from build123d import *

# Parameters (mm, degrees)
SKETCH_1_W          = 29.00004826
SKETCH_1_H          = 8.2
EXTRUDE_1_DEPTH     = 1
SKETCH_3_W          = 24.987345695
SKETCH_3_H          = 8.2
EXTRUDE_2_DEPTH     = 1
SKETCH_4_W          = 27.987350775
SKETCH_4_H          = 8.2
EXTRUDE_3_DEPTH     = 1
SKETCH_6_W          = 23.983586282
SKETCH_6_H          = 8.2
EXTRUDE_4_DEPTH     = 1
SKETCH_9_W          = 12.5
SKETCH_9_H          = 4.4
CUT_EXTRUDE_1_DEPTH = 1
SKETCH_10_W         = 29.00004826
SKETCH_10_H         = 25.974648209
EXTRUDE_5_DEPTH     = 1
SKETCH_11_W         = 13.604013208
SKETCH_11_H         = 7
CUT_EXTRUDE_3_DEPTH = 1
FILLET_1_R          = 1
FILLET_2_R          = 1
CUT_EXTRUDE_START   = -8.200051
SKETCH_12_W         = 27.27465329
SKETCH_12_H         = 24.274648209
SKETCH_12_W_2       = 26.97465329
SKETCH_12_H_2       = 23.974648209
CUT_EXTRUDE_4_DEPTH = 8.200051
EXTRUDE_START       = -5.1e-05
SKETCH_14_W         = 0.8
SKETCH_14_H         = 0.8
EXTRUDE_6_DEPTH     = 2
FILLET_3_R          = 0.8


# Some blends are built 0.0001 mm under size
with BuildPart() as part:
    # 草图1 → 凸台-拉伸1 (new body)
    with BuildSketch(Plane.XY):
        with Locations((-13.373026416, 0.4999492)):
            Rectangle(SKETCH_1_W, SKETCH_1_H)
    extrude(amount=EXTRUDE_1_DEPTH)

    # 草图3 → 凸台-拉伸2 (add)
    with BuildSketch(Plane.ZY.offset(26.860353061)):
        with Locations((-12.493672848, 0.4999492)):
            Rectangle(SKETCH_3_W, SKETCH_3_H)
    extrude(amount=EXTRUDE_2_DEPTH)

    # 草图4 → 凸台-拉伸3 (add)
    with BuildSketch(Plane(origin=(0, 0, -23.974648209), x_dir=(-1, 0, 0), z_dir=(0, 0, -1))):
        with Locations((12.866677673, 0.4999492)):
            Rectangle(SKETCH_4_W, SKETCH_4_H)
    extrude(amount=EXTRUDE_3_DEPTH)

    # 草图6 → 凸台-拉伸4 (add)
    with BuildSketch(Plane(origin=(0.114300229, 0, 0), x_dir=(0, 0, -1), z_dir=(1, 0, 0))):
        with Locations((11.991793141, 0.5)):
            Rectangle(SKETCH_6_W, SKETCH_6_H)
    extrude(amount=EXTRUDE_4_DEPTH)

    # 草图9 → 切除-拉伸1 (cut)
    with BuildSketch(Plane(origin=(1.114300229, 0, 0), x_dir=(0, 0, -1), z_dir=(1, 0, 0))):
        with Locations((11.541221742, 2.4)):
            Rectangle(SKETCH_9_W, SKETCH_9_H)
    extrude(amount=-CUT_EXTRUDE_1_DEPTH, mode=Mode.SUBTRACT)

    # 草图10 → 凸台-拉伸5 (add)
    with BuildSketch(Plane.XZ.offset(3.6)):
        with Locations((-13.373026416, -11.987324105)):
            Rectangle(SKETCH_10_W, SKETCH_10_H)
    extrude(amount=EXTRUDE_5_DEPTH)

    # 草图11 → 切除-拉伸3 (cut)
    with BuildSketch(Plane.XZ.offset(4.6)):
        with Locations((-15.621031242, -16.494333249)):
            Rectangle(SKETCH_11_W, SKETCH_11_H)
    extrude(amount=-CUT_EXTRUDE_3_DEPTH, mode=Mode.SUBTRACT)

    # 圆角1
    fillet_1_edges = [part.edges().sort_by_distance(p)[0] for p in [
        (1.126997714, -2.54e-05, -24.974648209),
        (1.126997714, -2.54e-05, 1),
        (-27.873050546, -2.54e-05, 1),
        (-27.873050546, -4.1, -24.974648209),
    ]]
    fillet(fillet_1_edges, radius=FILLET_1_R)

    # 圆角2
    fillet_2_edges = [part.edges().sort_by_distance(p)[0] for p in [
        (-27.860353061, 0.4999492, -24.987345695),
    ]]
    fillet(fillet_2_edges, radius=FILLET_2_R - 0.0001)  # a hair under: the kernel refuses the full size

    # 草图12 → 切除-拉伸4 (cut)
    with BuildSketch(Plane(origin=(0, 4.6, 0), x_dir=(1, 0, 0), z_dir=(0, 1, 0)).offset(CUT_EXTRUDE_START)):
        with Locations((-13.373026416, 11.987324105)):
            Rectangle(SKETCH_12_W, SKETCH_12_H)
        with Locations((-13.373026416, 11.987324105)):
            Rectangle(SKETCH_12_W_2, SKETCH_12_H_2, mode=Mode.SUBTRACT)
    extrude(amount=CUT_EXTRUDE_4_DEPTH, mode=Mode.SUBTRACT)

    # 草图14 → 凸台-拉伸6 (add)
    with BuildSketch(Plane(origin=(0, -3.6, 0), x_dir=(1, 0, 0), z_dir=(0, 1, 0)).offset(EXTRUDE_START)):
        with Locations((-26.610353061, 23.724648209)):
            Rectangle(SKETCH_14_W, SKETCH_14_H)
        with Locations((-0.135699771, 0.25)):
            Rectangle(SKETCH_14_W, SKETCH_14_H)
    extrude(amount=EXTRUDE_6_DEPTH)

    # 圆角3
    # the kernel refuses this fillet: 0.8 mm, written as the material it adds along each edge
    with BuildSketch(Plane(origin=(-27.010353061, -3.600051, 0.15), x_dir=(0, 0, -1), z_dir=(0, 1, 0)), Plane(origin=(-27.010353061, -3.600051, -24.124648209), x_dir=(1, 0, 0), z_dir=(0, 1, 0))) as fillet_3_piece_1:
        with BuildLine():
            CenterArc((FILLET_3_R, -FILLET_3_R), FILLET_3_R, 90, 90)
            Line((0, -FILLET_3_R), (0, 0))
            Line((0, 0), (FILLET_3_R, 0))
        make_face()
    extrude(amount=8.2000002)
    with BuildSketch(Plane(origin=(0.264300229, -3.600051, 0.15), x_dir=(0, 0, -1), z_dir=(0, 1, 0))) as fillet_3_piece_2_section:
        with BuildLine():
            CenterArc((FILLET_3_R, FILLET_3_R), FILLET_3_R, 180, 90)
            Line((0, FILLET_3_R), (0, 0))
            Line((0, 0), (FILLET_3_R, 0))
        make_face()
    fillet_3_piece_2 = extrude(amount=10.2000002, mode=Mode.PRIVATE)
    fillet_3_piece_2 = split(fillet_3_piece_2, bisect_by=Plane(origin=(0.183426008, 4.6, -0.178427163), z_dir=(0, -1, 0)), keep=Keep.TOP, mode=Mode.PRIVATE)
    add(fillet_3_piece_2)
    with BuildSketch(Plane(origin=(0.264300229, -3.600051, -24.124648209), x_dir=(0, 0, 1), z_dir=(0, 1, 0))) as fillet_3_piece_3_section:
        with BuildLine():
            CenterArc((FILLET_3_R, -FILLET_3_R), FILLET_3_R, 90, 90)
            Line((0, -FILLET_3_R), (0, 0))
            Line((0, 0), (FILLET_3_R, 0))
        make_face()
    fillet_3_piece_3 = extrude(amount=10.2000002, mode=Mode.PRIVATE)
    fillet_3_piece_3 = split(fillet_3_piece_3, bisect_by=Plane(origin=(0.180139074, 4.6, -23.803633202), z_dir=(0, -1, 0)), keep=Keep.TOP, mode=Mode.PRIVATE)
    add(fillet_3_piece_3)


solid = part.part
Design review of the part built by this model. Coordinates are the model's own, in mm. A direction names the side the tool comes from. Coordinates: 2 decimals unless noted, no trailing zeros. Order: outer loops, then holes, each group sorted by start corner. A loop starts at its lowest first (then second) coordinate and runs counter-clockwise, first axis right, second up. Notation, with made-up numbers: (-1.75, 30) -> (52.25, 30) arc R16 ccw to (52.25, 48) -> close; hole circle Ø8 at (3.25, 6). An arc over 180 degrees is marked (long way). Use one line per item in the form item = value. Start each with the question number.
(1) For probe 1 along X at (y, z) = (-2, -21); probe 2 along Z at (x, y) = (-4.75, -1), list the stretches that pass through material, from the lowest coordinate up.
(2) For faces 1 (the flat face through (0.7, 2.4, -5.291)), 2 (the cylindrical face through (0.024, 1.457, -0.078)), 3 (the flat face through (-22.423, -4, -17)), list the 3-axis set-ups (+Z, -Z, +X, -X, +Y, -Y) from which the entire face can be reached by the end or side of a thin tool; tool diameter is ignored.
(3) Add section B-B on y = -4. State the section outline as (x, z) points, plus the area to 3 significant figures.
(4) The part is to be moulded in two halves that separate along X. For faces 4 (the flat face through (-26.5, -1.6, -23.6)), 5 (the flat face through (0.7, 2.4, -17.791)), 6 (the flat face through (1.127, -4, -12)), 7 (the cylindrical face through (-27.56, 0.56, -24.7)), say which applies: +X half, -X half, draft (parallel to the pull), parting line (faces both ways), or undercut.
(5) Insertion check: pin 1 (6 mm diameter, centred on x = -24.5, z = -11, fed in from +Y); pin 2 (2 mm diameter, centred on x = -16.5, y = 1, fed in from -Z); pin 3 (0.7 mm diameter, centred on x = 1, y = 2, fed in from -Z); pin 4 (1 mm diameter, centred on y = -1, z = -21, fed in from +X). Each pin has a flat end and moves straight along its axis. Give the tip position at first contact, or say it passes through.
Answer block:
q1.probe_1 = -27.86 to -27.01, 0.26 to 1.11
q1.probe_2 = -24.97 to -24.12, 0.15 to 1
q2.face_1 = +X, +Y
q2.face_2 = +Y
q2.face_3 = +Y, -Y
q3.outline = (-27.87, -23.97) arc R1 ccw to (-26.87, -24.97) -> (0.13, -24.97) arc R1 ccw to (1.13, -23.97) -> (1.13, 0) arc R1 ccw to (0.13, 1) -> (-26.87, 1) arc R1 ccw to (-27.87, 0) -> close; hole (-22.42, -19.99) -> (-8.82, -19.99) -> (-8.82, -12.99) -> (-22.42, -12.99) -> close
q3.area = 657 mm²
q4.face_4 = undercut
q4.face_5 = draft
q4.face_6 = +X half
q4.face_7 = -X half
q5.pin_1 = 4.6
q5.pin_2 = -24.97
q5.pin_3 = -24.83
q5.pin_4 = 1.11
